Source: CAD feature listing. Evaluate the final solid. Frame: model axes, mm. Face numbers are marked on the shaded views. A direction names the side the tool comes from. Round coordinates to 2 decimals unless told otherwise and drop trailing zeros. Order: outer loops, then holes, each group sorted by start corner. A loop starts at its lowest first (then second) coordinate and runs counter-clockwise, first axis right, second up. Notation, with made-up numbers: M 4.25,-35.5 L 21.25,-35.5 A18 cw 21.25,-12.5 Z; hole C 89.5,40.25 d1. An arc over 180 degrees is marked long. Use one line per item in the form item = value. Start each with the question number.
Q1. Section A-A (z = 0). Return the cut outline in (x, y), plus the area to 4 significant figures.
Q2. Section B-B (x = 0). Return the cut outline in (y, z).
Q3. Reachability of the marked faces 1, 2, 3 and 4 from +Z, -Z, +X, -X, +Y, -Y: full face, straight path, thin tool, end or side. Return the list, or none.
Q4. Section C-C (y = 1). Return the cut outline in (x, z), plus the area to 3 significant figures.
Q5. Material intervals for probe 1 along Y at (x, z) = (3, 0); probe 2 along Z at (x, y) = (2, 3); probe 3 along Z at (x, y) = (0, 2.5), sorted ascending.
Q6. Section D-D (y = 6.5). Return the cut outline in (x, z), plus the area to 3 significant figures.
Q7. Contact query for flat-ended pins moving along their axis: pin 1 (1 mm diameter, centred on y = 7.5, z = 1.5, fed in from -X); pin 2 (4 mm diameter, centred on x = 1.5, z = -1, fed in from -Y); pin 3 (1 mm diameter, centred on x = 1, y = 7, fed in from -Z); pin 4 (1.2 mm diameter, centred on x = 0.5, y = 7, fed in from +Z). Output: stop coordinate, or through.
from build123d import *
from build123d.topology import SkipClean

# Parameters (mm, degrees)
SKETCH_1_R      = 4
EXTRUDE_1_DEPTH = 1.5
SKETCH_3_R      = 2.5
EXTRUDE_3_DEPTH = 2
EXTRUDE_2_DEPTH = 6
CHAMFER_1_SIZE  = 0.5


with BuildPart() as part:
    # 草图1 → 凸台-拉伸1 (new body)
    with BuildSketch(Plane(origin=(0, 0, 0), x_dir=(1, 0, 0), z_dir=(0, 1, 0))):
        with Locations(Location((0, 0, 0), (0, 0, 270))):
            Circle(SKETCH_1_R)
    extrude(amount=EXTRUDE_1_DEPTH)

    # 草图3 → 凸台-拉伸3 (add)
    with BuildSketch(Plane(origin=(0, 1.5, 0), x_dir=(1, 0, 0), z_dir=(0, 1, 0))):
        with Locations(Location((0, 0, 0), (0, 0, 270))):
            Circle(SKETCH_3_R)
    extrude(amount=EXTRUDE_3_DEPTH)

    # 草图2 → 凸台-拉伸2 (add)
    with SkipClean():  # the faces are left unmerged after this step: merging them gives an invalid solid
        with BuildSketch(Plane(origin=(0, 3.5, 0), x_dir=(1, 0, 0), z_dir=(0, 1, 0))):
            with BuildLine():
                Line((-2, 1.5), (2, 1.5))
                ThreePointArc((2, 1.5), (2.5, 0), (2, -1.5))
                Line((2, -1.5), (-2, -1.5))
                ThreePointArc((-2, -1.5), (-2.5, 0), (-2, 1.5))
            make_face()
        extrude(amount=EXTRUDE_2_DEPTH)

    # 倒角1
    chamfer_1_edges = [part.edges().sort_by_distance(p)[0] for p in [
        (-2.5, 9.5, 0),
        (2.5, 9.5, 0),
    ]]
    chamfer(chamfer_1_edges, length=CHAMFER_1_SIZE)


solid = part.part
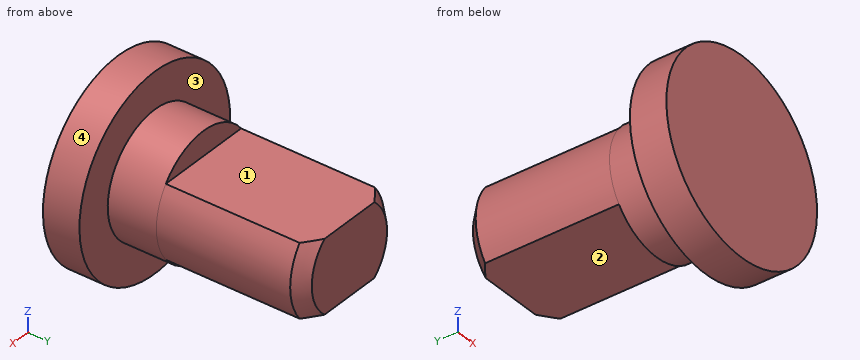
Results list:
q1.outline = M -4,0 L 4,0 L 4,1.5 L 2.5,1.5 L 2.5,9 L 2,9.5 L -2,9.5 L -2.5,9 L -2.5,1.5 L -4,1.5 Z
q1.area = 51.75 mm2
q2.outline = M 0,-4 L 1.5,-4 L 1.5,-2.5 L 3.5,-2.5 L 3.5,-1.5 L 9.5,-1.5 L 9.5,1.5 L 3.5,1.5 L 3.5,2.5 L 1.5,2.5 L 1.5,4 L 0,4 Z
q3.face_1 = +Z, +X, -X, +Y
q3.face_2 = -Z, +X, -X, +Y
q3.face_3 = +Y
q3.face_4 = +Y, -Y
q4.outline = C 0,0 d8
q4.area = 50.3 mm2
q5.probe_1 = 0 to 1.5
q5.probe_2 = -1.5 to 1.5
q5.probe_3 = -2.5 to 2.5
q6.outline = M -2,-1.5 L 2,-1.5 A2.5 ccw 2,1.5 L -2,1.5 A2.5 ccw Z
q6.area = 14.0 mm2
q7.pin_1 = -2.29
q7.pin_2 = 0
q7.pin_3 = -1.5
q7.pin_4 = 1.5
